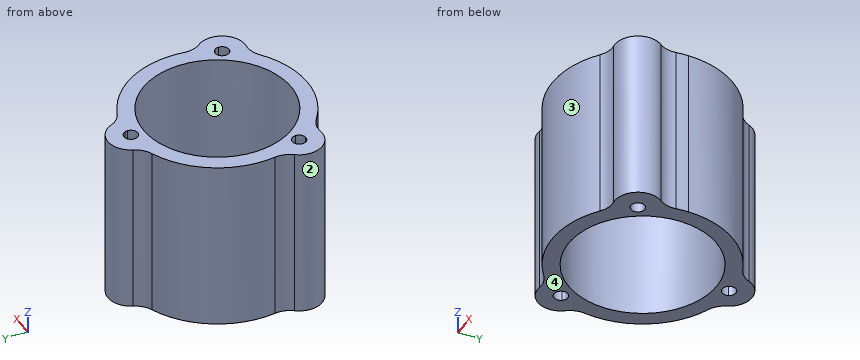
from build123d import *

# Parameters (mm, degrees)
F0_R     = 20.32
F1_DEPTH = 47.625
F2_R     = 6.35


with BuildPart() as f1:
    # F0 (on Top) → F1 (new body)
    with BuildSketch(Plane.XY):
        with BuildLine():
            ThreePointArc((23.9050999455, -6.4692674698), (24.5490837421, -3.2630832697), (24.765, 0))
            ThreePointArc((24.765, 0), (19.6285885254, 15.1004548773), (6.35, 23.9370575677))
            ThreePointArc((6.35, 23.9370575677), (4.0651088886, 24.4290833787), (1.7440091422, 24.703515076))
            ThreePointArc((1.7440091422, 24.703515076), (1.8643178935, 24.3286489263), (1.905, 23.9370575677))
            ThreePointArc((1.905, 23.9370575677), (-0.3915913586, 22.0727396742), (-1.7440091422, 24.703515076))
            ThreePointArc((-1.7440091422, 24.703515076), (-4.0651088886, 24.4290833787), (-6.35, 23.9370575677))
            ThreePointArc((-6.35, 23.9370575677), (-21.4471191247, 12.3825), (-23.9050999455, -6.4692674698))
            ThreePointArc((-23.9050999455, -6.4692674698), (-23.1887612414, -8.6940541227), (-22.2658761897, -10.8414013165))
            ThreePointArc((-22.2658761897, -10.8414013165), (-20.1370690632, -10.1581864481), (-18.8250999455, -11.9685287839))
            ThreePointArc((-18.8250999455, -11.9685287839), (-19.3113489683, -13.239815795), (-20.5218670475, -13.8621137596))
            ThreePointArc((-20.5218670475, -13.8621137596), (-19.1236523528, -15.735029256), (-17.5550999455, -17.4677900979))
            ThreePointArc((-17.5550999455, -17.4677900979), (0, -24.765), (17.5550999455, -17.4677900979))
            ThreePointArc((17.5550999455, -17.4677900979), (19.1236523528, -15.735029256), (20.5218670475, -13.8621137596))
            ThreePointArc((20.5218670475, -13.8621137596), (19.0803215513, -11.0160287839), (22.2658761897, -10.8414013165))
            ThreePointArc((22.2658761897, -10.8414013165), (23.1887612414, -8.6940541227), (23.9050999455, -6.4692674698))
        make_face()
        Circle(F0_R, mode=Mode.SUBTRACT)
        with BuildLine():
            ThreePointArc((-22.2658761897, -10.8414013165), (-23.1887612414, -8.6940541227), (-23.9050999455, -6.4692674698))
            ThreePointArc((-23.9050999455, -6.4692674698), (-26.2293612595, -15.1435287839), (-17.5550999455, -17.4677900979))
            ThreePointArc((-17.5550999455, -17.4677900979), (-19.1236523528, -15.735029256), (-20.5218670475, -13.8621137596))
            ThreePointArc((-20.5218670475, -13.8621137596), (-22.3798783397, -12.9210287839), (-22.2658761897, -10.8414013165))
        make_face()
        with BuildLine():
            ThreePointArc((1.7440091422, 24.703515076), (4.0651088886, 24.4290833787), (6.35, 23.9370575677))
            ThreePointArc((6.35, 23.9370575677), (0, 30.2870575677), (-6.35, 23.9370575677))
            ThreePointArc((-6.35, 23.9370575677), (-4.0651088886, 24.4290833787), (-1.7440091422, 24.703515076))
            ThreePointArc((-1.7440091422, 24.703515076), (0, 25.8420575677), (1.7440091422, 24.703515076))
        make_face()
        with BuildLine():
            ThreePointArc((17.5550999455, -17.4677900979), (26.2293612595, -15.1435287839), (23.9050999455, -6.4692674698))
            ThreePointArc((23.9050999455, -6.4692674698), (23.1887612414, -8.6940541227), (22.2658761897, -10.8414013165))
            ThreePointArc((22.2658761897, -10.8414013165), (22.5404422812, -11.3754979015), (22.6350999455, -11.9685287839))
            ThreePointArc((22.6350999455, -11.9685287839), (22.0013869566, -13.3872797611), (20.5218670475, -13.8621137596))
            ThreePointArc((20.5218670475, -13.8621137596), (19.1236523528, -15.735029256), (17.5550999455, -17.4677900979))
        make_face()
    extrude(amount=F1_DEPTH)

    # F2
    f2_edges = [f1.edges().sort_by_distance(p)[0] for p in [
        (6.35, 23.937058, 23.8125),
        (-23.9051, -6.469267, 23.8125),
        (17.5551, -17.46779, 23.8125),
        (23.9051, -6.469267, 23.8125),
        (-6.35, 23.937058, 23.8125),
        (-17.5551, -17.46779, 23.8125),
    ]]
    fillet(f2_edges, radius=F2_R)


solid = f1.part
Verification items for the finished model (mm, model axes). Face numbers are marked on the shaded views. Coordinates: 2 decimals unless noted, no trailing zeros. Loops run counter-clockwise (first coordinate to the right, second up) from the corner with the lowest first, then second, coordinate; pieces in that order, holes last. Notation, with made-up numbers: (48, -22) -> (54, -22) arc R31 ccw to (54, 16) -> close; hole circle Ø7 at (37, 41.25). An arc over 180 degrees is marked (long way). Write each question's results on one line, items separated by ' | '.
Item 1: Mould release check, pull along Y, two halves, no side actions. Record for the marked faces 1, 2, 3 and 4: +Y half, -Y half, draft (parallel to the pull), parting line (faces both ways), or undercut.
Found:
face 1: undercut | face 2: parting line | face 3: -Y half | face 4: draft
Item 2: Section check D-D, the plane z = 39.5. Count the separate pieces of the cut face and the enclosed holes in it, plus the area to 3 significant figures.
Found:
separate pieces: 1 | enclosed holes: 4 | area: 773 mm2
Item 3: Gauge pin test, flat ends, axial feed: pin 1 (1.5 mm diameter, centred on x = 16.5, z = 37.5, fed in from +Y); pin 2 (10 mm diameter, centred on x = 16.5, z = 14, fed in from +Y); pin 3 (8 mm diameter, centred on x = -10.5, z = 36.5, fed in from +Y). Record the tip position at first contact, or that the pin passes through.
Found:
pin 1: stops at y = 19.11 | pin 2: stops at y = 21.93 | pin 3: stops at y = 25.21
Item 4: Section check A-A, the plane x = 0. Enter the section's corners in (y, z) (3 decimals), plus the area to 3 significant figures.
Found:
outline: (-24.765, 0) -> (-20.32, 0) -> (-20.32, 47.625) -> (-24.765, 47.625) -> close; (20.32, 0) -> (22.032, 0) -> (22.032, 47.625) -> (20.32, 47.625) -> close; (25.842, 0) -> (30.287, 0) -> (30.287, 47.625) -> (25.842, 47.625) -> close | area: 505 mm2
Item 5: Section check B-B, the plane x = 10.5. Enter the section's corners in (y, z) (3 decimals).
Found:
outline: (-22.429, 0) -> (-17.397, 0) -> (-17.397, 47.625) -> (-22.429, 47.625) -> close; (17.397, 0) -> (22.429, 0) -> (22.429, 47.625) -> (17.397, 47.625) -> close
Item 6: Section check C-C, the plane y = 7.5. Enter the section's corners in (x, z) (3 decimals).
Found:
outline: (-23.602, 0) -> (-18.885, 0) -> (-18.885, 47.625) -> (-23.602, 47.625) -> close; (18.885, 0) -> (23.602, 0) -> (23.602, 47.625) -> (18.885, 47.625) -> close
Item 7: Material ranges on L1, parallel to X at y = 14, z = 31.5; L2, parallel to X at y = 9.5, z = 9; L3, parallel to Y at x = -11.5, z = 15.5, recorded low to high.
Found:
L1: x = -20.43 to -14.73, 14.73 to 20.43 | L2: x = -22.87 to -17.96, 17.96 to 22.87 | L3: y = -21.93 to -16.75, 16.75 to 21.93
